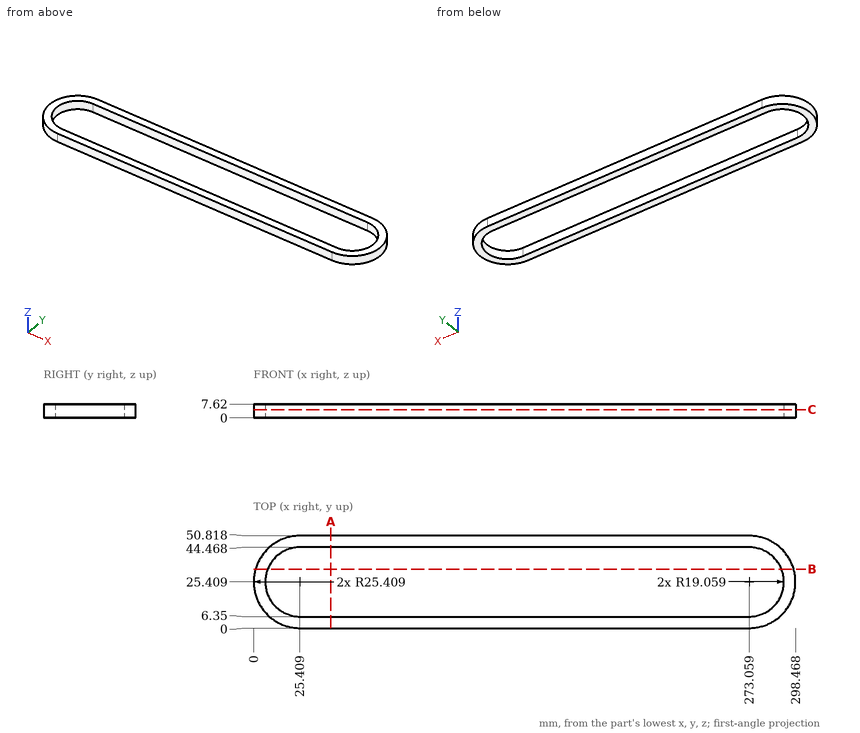
The figure shows three views and two pictorial views of one solid part (mm, origin at its lowest corner). Answer the questions. Coordinates: 2 decimals unless noted, no trailing zeros. Loops run counter-clockwise (first coordinate to the right, second up) from the corner with the lowest first, then second, coordinate; pieces in that order, holes last.
1) Find section B-B on y = 32.5. Write down the section's boundary in (x, z), then the cut area to 3 significant figures.
2) Find section A-A on x = 42.5. Write down the section's boundary in (y, z), then the cut area to 3 significant figures.
3) Flat-ended cylindrical pins translate along their axes: pin 1 Ø4 at (y, z) = (35.5, 1.5) entering from -X; pin 2 Ø1.5 at (y, z) = (43, 6) entering from +X (1 decimal); pin 3 Ø1.5 at (y, z) = (19, 4.5) entering from +X. Find the tip coordinate at first contact, or state that the pin passes through.
4) Find the intervals of material crossed by L1, parallel to Y at x = 177, z = 3.25; L2, parallel to X at y = 26, z = 2.75; L3, parallel to X at y = 12.5, z = 5.5 (1 decimal), in increasing order.
5) Find section C-C on z = 4.5. Write down the section's boundary in (x, y), then the cut area to 3 significant figures.
Values:
1. outline: (1.01, 0) - (7.72, 0) - (7.72, 7.62) - (1.01, 7.62) - close; (290.75, 0) - (297.46, 0) - (297.46, 7.62) - (290.75, 7.62) - close
1. area: 102 mm2
2. outline: (0, 0) - (6.35, 0) - (6.35, 7.62) - (0, 7.62) - close; (44.47, 0) - (50.82, 0) - (50.82, 7.62) - (44.47, 7.62) - close
2. area: 96.8 mm2
3. pin 1: stops at x = 1.32
3. pin 2: stops at x = 292.1
3. pin 3: stops at x = 297.83
4. L1: y = 0 to 6.35, 44.47 to 50.82
4. L2: x = 0.01 to 6.36, 292.11 to 298.46
4. L3: x = 3.5 to 11.4, 287.1 to 294.9
5. outline: (25.41, 0) - (273.06, 0) arc R25.41 ccw to (273.06, 50.82) - (25.41, 50.82) arc R25.41 ccw to start; hole (25.41, 6.35) - (273.06, 6.35) arc R19.06 ccw to (273.06, 44.47) - (25.41, 44.47) arc R19.06 ccw to start
5. area: 4,030 mm2
